Check sheet for the modelled part. Datum: model origin and axes. Units: mm. Face numbers are marked on the shaded views. Give positions to 0.01 mm unless a question says otherwise; leave off trailing zeros. Loops run counter-clockwise (first coordinate to the right, second up) from the corner with the lowest first, then second, coordinate; pieces in that order, holes last. Notation, with made-up numbers: (70, -38.75) - (102, -38.75) arc R19 cw to (102, -32.75) - close; hole circle Ø3 at (80.25, 65). An arc over 180 degrees is marked (long way). Use one line per item in the form item = value.
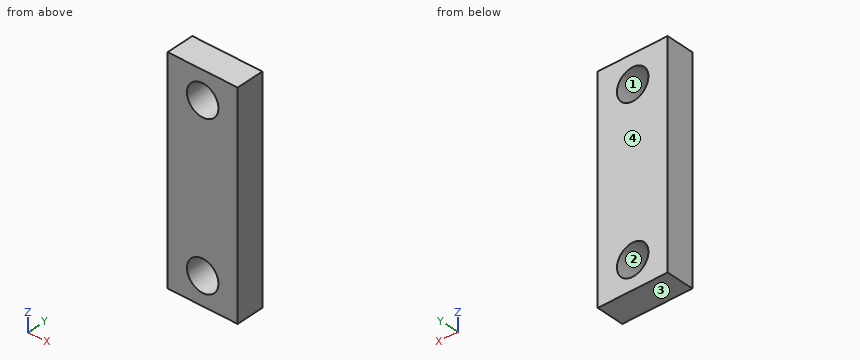
Autodesk Inventor part; units mm, degrees
ref_plane "Work Plane1" through (0, 0, 15.5) normal (0, 0, 1) x (1, 0, 0)
ref_plane "YZ Plane" through (0, 0, 0) normal (1, 0, 0) x (0, 1, 0)
ref_plane "XZ Plane" through (0, 0, 0) normal (0, 1, 0) x (-1, 0, 0)
ref_plane "Work Plane1" through (0, 0, 15.5) normal (0, 0, 1) x (1, 0, 0)
sketch "Sketch1" plane through (0, 0, 15.5) normal (0, 0, 1) x (1, 0, 0)
  line L0 (5, 4) -> (5, 0)
  line L1 (-5, 4) -> (5, 4)
  line L2 (-5, 0) -> (5, 0)
  line L3 (-5, 4) -> (-5, 0)
extrude "Extrusion1" add sketch "Sketch1" against normal blind 31
hole "Hole2" at (0, 4, -11.5) direction (0, -1, 0) diameter 4.5 depth 4
sketch "Sketch2" plane through (-5, 4, 15.5) normal (0, 1, 0) x (1, 0, 0)
  point P0 (5, 27)
hole "Hole1" at (0, 4, 11.5) direction (0, -1, 0) diameter 4.5 depth 4
sketch "Sketch3" plane through (-5, 4, 15.5) normal (0, 1, 0) x (1, 0, 0)
  point P0 (5, 4)
properties part number "Spreader Belt clamp" material "ASA Plastic"
Item 1: Gauge pin test, flat end, axial feed: P1, Ø5, axis at x = 3, z = 12, coming from the -Y side. Record the tip position at first contact, or that the pin passes through.
Answer block:
P1 = 0
Item 2: Thickness scan on L1, parallel to Z at x = 0, y = 2.25; L2, parallel to X at y = 2.7, z = -11.5; L3, parallel to Z at x = 2, y = 3.6. Record the ranges inside material, lowest first.
Answer block:
L1 = -15.5 to -13.75, -9.25 to 9.25, 13.75 to 15.5
L2 = -5 to -2.25, 2.25 to 5
L3 = -15.5 to -12.53, -10.47 to 10.47, 12.53 to 15.5
Item 3: Section check A-A on z = 11.5. Record the boundary of the cut face in (x, y).
Answer block:
outline = (-5, 0) - (-2.25, 0) - (-2.25, 4) - (-5, 4) - close; (2.25, 0) - (5, 0) - (5, 4) - (2.25, 4) - close
Item 4: Section check C-C on x = 0. Record the boundary of the cut face in (y, z).
Answer block:
outline = (0, -15.5) - (4, -15.5) - (4, -13.75) - (0, -13.75) - close; (0, -9.25) - (4, -9.25) - (4, 9.25) - (0, 9.25) - close; (0, 13.75) - (4, 13.75) - (4, 15.5) - (0, 15.5) - close
Item 5: Mould release check, pull along Z, two halves, no side actions. Record for the marked faces 1, 2, 3 and 4: released by +Z, released by -Z, zero draft, split by the parting line, or undercut.
Answer block:
face_1 = undercut
face_2 = undercut
face_3 = released by -Z
face_4 = zero draft
Item 6: Section check B-B on y = 2.5. Record the boundary of the cut face in (x, z).
Answer block:
outline = (-5, -15.5) - (5, -15.5) - (5, 15.5) - (-5, 15.5) - close; hole circle Ø4.5 at (0, -11.5); hole circle Ø4.5 at (0, 11.5)
Item 7: Section check D-D on x = -1.75. Record the boundary of the cut face in (y, z), then the cut area to 3 significant figures.
Answer block:
outline = (0, -15.5) - (4, -15.5) - (4, -12.91) - (0, -12.91) - close; (0, -10.09) - (4, -10.09) - (4, 10.09) - (0, 10.09) - close; (0, 12.91) - (4, 12.91) - (4, 15.5) - (0, 15.5) - close
area = 101 mm2
